from build123d import *

# Parameters (mm, degrees)
CROQUIS1_R                   = 15.000000000000002
SALIENTE_EXTRUIR1_DEPTH      = 8
CROQUIS2_R                   = 4.000000000000007
CROQUIS2_R_2                 = 1.4999999999999973
CORTAR_EXTRUIR1_DEPTH        = 3
SALIENTE_EXTRUIR2_START      = -4
SALIENTE_EXTRUIR2_DEPTH      = 4
SALIENTE_EXTRUIR3_DEPTH      = 10
SALIENTE_EXTRUIR3_DEPTH_BACK = 10
CROQUIS4_R                   = 1.999999999999995
CORTAR_EXTRUIR2_DEPTH        = 26.000000000000004
CROQUIS6_R                   = 1.499999999999999
CORTAR_EXTRUIR3_DEPTH        = 0.5


with BuildPart() as part:
    # Croquis1 → Saliente-Extruir1 (new body)
    with BuildSketch(Plane(origin=(3.102503887066035, -26.412068884743757, 0.2313913751144545), x_dir=(0.9931720445250996, 0.11665438489091776, -0.0010219880408017562), z_dir=(0.11665886153153528, -0.9931339327669669, 0.008700667387268338))):
        with Locations(Location((-115.80198834358447, 158.9846336736222, 0), (0, 0, 0.058557828))):
            Circle(CROQUIS1_R)
    extrude(amount=SALIENTE_EXTRUIR1_DEPTH)

    # Croquis2 → Cortar-Extruir1 (cut)
    with BuildSketch(Plane(origin=(4.03577477931832, -34.35714034687951, 0.3009967142126015), x_dir=(0.9931720445250996, 0.11665438489091778, -0.0010219880408017569), z_dir=(0.1166588615315353, -0.9931339327669669, 0.00870066738726834))):
        with Locations(Location((-115.8019883435845, 158.9846336736222, 0), (0, 0, 0.058557828))):
            Circle(CROQUIS2_R)
        with Locations(Location((-115.8019883435845, 168.9846336736222, 0), (0, 0, 0.058557828))):
            Circle(CROQUIS2_R_2)
        with Locations(Location((-115.8019883435845, 148.9846336736222, 0), (0, 0, 0.058557828))):
            Circle(CROQUIS2_R_2)
    extrude(amount=-CORTAR_EXTRUIR1_DEPTH, mode=Mode.SUBTRACT)

    # Croquis3 → Saliente-Extruir2 (add)
    with BuildSketch(Plane(origin=(4.03577477931832, -34.35714034687951, 0.3009967142126015), x_dir=(0.9931720445250996, 0.11665438489091778, -0.0010219880408017569), z_dir=(0.1166588615315353, -0.9931339327669669, 0.00870066738726834)).offset(SALIENTE_EXTRUIR2_START)):
        with BuildLine():
            Line((-140.80198834358453, 161.9846336736222), (-130.49892680028356, 161.9846336736222))
            ThreePointArc((-130.49892680028356, 161.98463367362223), (-129.9260267482204, 164.03552855912218), (-129.06848750500595, 165.98463367362243))
            Line((-129.0684875050059, 165.9846336736222), (-140.80198834358453, 165.9846336736222))
            Line((-140.80198834358453, 165.9846336736222), (-140.80198834358453, 161.9846336736222))
        make_face()
        with BuildLine():
            ThreePointArc((-129.06848750500598, 151.98463367362197), (-129.9260267482204, 153.9337387881222), (-130.49892680028356, 155.98463367362217))
            Line((-130.49892680028356, 155.9846336736222), (-140.80198834358453, 155.9846336736222))
            Line((-140.80198834358453, 155.9846336736222), (-140.80198834358453, 151.9846336736222))
            Line((-140.80198834358453, 151.9846336736222), (-129.06848750500592, 151.9846336736222))
        make_face()
        with BuildLine():
            Line((-125.01691169330087, 151.9846336736222), (-125.01691169330087, 155.9846336736222))
            Line((-125.01691169330087, 155.9846336736222), (-130.49892680028356, 155.9846336736222))
            ThreePointArc((-130.49892680028356, 155.98463367362217), (-129.9260267482204, 153.9337387881222), (-129.06848750500598, 151.98463367362197))
            Line((-129.06848750500592, 151.9846336736222), (-125.01691169330087, 151.9846336736222))
        make_face()
        with BuildLine():
            Line((-130.49892680028356, 161.9846336736222), (-125.01691169330087, 161.9846336736222))
            Line((-125.01691169330087, 161.9846336736222), (-125.01691169330087, 165.9846336736222))
            Line((-125.01691169330087, 165.9846336736222), (-129.0684875050059, 165.9846336736222))
            ThreePointArc((-129.06848750500595, 165.98463367362243), (-129.9260267482204, 164.03552855912218), (-130.49892680028356, 161.98463367362223))
        make_face()
    extrude(amount=SALIENTE_EXTRUIR2_DEPTH)

    # Croquis4 → Saliente-Extruir3 (add, two sides: drawn at the far end of the back side and taken through both)
    with BuildSketch(Plane(origin=(-6.683e-14, 1.3927822726245929, 158.97853283345188), x_dir=(1, 0, 4.2e-16), z_dir=(0, 0.008760483579084877, 0.9999616262274571)).offset(-SALIENTE_EXTRUIR3_DEPTH_BACK)):
        with Locations(Location((-134.05179749109138, -48.5645966599886, 0), (0, 0, 276.699314902))):
            Circle(CROQUIS4_R)
    extrude(amount=SALIENTE_EXTRUIR3_DEPTH + SALIENTE_EXTRUIR3_DEPTH_BACK)

    # Croquis5 → Cortar-Extruir2 (cut)
    with BuildSketch(Plane(origin=(-7.073e-14, 1.4803871084154419, 168.97814909572648), x_dir=(1, 0, 4.2e-16), z_dir=(0, 0.008760483579084877, 0.9999616262274571))):
        Polygon((-137.1921048729679, -53.52505022011607), (-133.51980518703422, -53.09369867037679), (-133.8184797680283, -50.5509407490388), (-135.80482385707867, -50.78425847210188), (-136.03814158014168, -48.79791438305168), (-136.2714593032048, -46.81157029400149), (-134.28511521415442, -46.578252570938396), (-134.47954467160224, -44.922982673441965), (-138.15184435753594, -45.35433422318124), align=None)
        with BuildLine():
            ThreePointArc((-136.03814158014154, -48.79791438305167), (-135.62133541037747, -47.32501982900029), (-134.28511521415442, -46.57825257093841))
            Line((-134.28511521415442, -46.578252570938396), (-136.2714593032048, -46.81157029400149))
            Line((-136.2714593032048, -46.81157029400149), (-136.03814158014168, -48.79791438305168))
        make_face()
        with BuildLine():
            ThreePointArc((-133.8184797680283, -50.550940749038816), (-135.2913743220797, -50.13413457927471), (-136.03814158014154, -48.79791438305167))
            Line((-136.03814158014168, -48.79791438305168), (-135.80482385707867, -50.78425847210188))
            Line((-135.80482385707867, -50.78425847210188), (-133.8184797680283, -50.5509407490388))
        make_face()
    extrude(amount=-CORTAR_EXTRUIR2_DEPTH, mode=Mode.SUBTRACT)

    # Croquis6 → Cortar-Extruir3 (cut)
    # profile 1 of 2: a face of its own
    with BuildSketch(Plane(origin=(4.03577477931832, -34.35714034687951, 0.3009967142126015), x_dir=(0.9931720445250996, 0.11665438489091778, -0.0010219880408017569), z_dir=(0.1166588615315353, -0.9931339327669669, 0.008700667387268341))):
        with BuildLine():
            Line((-111.32985238858495, 159.4846336736222), (-101.81091976395129, 159.4846336736222))
            ThreePointArc((-101.81091976395126, 159.48463367362265), (-112.97131478814173, 172.6954792792921), (-128.45109898425804, 164.9846336736222))
            Line((-128.45109898425804, 164.9846336736222), (-137.80198834358436, 164.98463367362217))
            Line((-137.80198834358436, 164.98463367362217), (-137.80198834358436, 162.98463367362217))
            Line((-137.80198834358436, 162.98463367362217), (-129.21839620858324, 162.9846336736222))
            ThreePointArc((-129.21839620858324, 162.9846336736222), (-129.6170142670406, 161.25290586501285), (-129.7930569232177, 159.48463367362226))
            Line((-129.7930569232177, 159.4846336736222), (-120.27412429858411, 159.4846336736222))
            ThreePointArc((-120.27412429858411, 159.48463367362217), (-115.80198834358455, 163.4846336736222), (-111.32985238858495, 159.48463367362223))
        make_face()
        with Locations(Location((-115.80198834358454, 168.9846336736222, 0), (0, 0, 0.058557828))):
            Circle(CROQUIS6_R, mode=Mode.SUBTRACT)
    # profile 2 of 2: a face of its own
    with BuildSketch(Plane(origin=(4.03577477931832, -34.35714034687951, 0.3009967142126015), x_dir=(0.9931720445250996, 0.11665438489091778, -0.0010219880408017569), z_dir=(0.1166588615315353, -0.9931339327669669, 0.008700667387268341))):
        with BuildLine():
            ThreePointArc((-128.45109898425804, 152.9846336736222), (-112.97131478814173, 145.2737880679523), (-101.81091976395126, 158.48463367362174))
            Line((-101.81091976395128, 158.4846336736222), (-111.32985238858495, 158.4846336736222))
            ThreePointArc((-111.32985238858495, 158.48463367362217), (-115.80198834358455, 154.4846336736222), (-120.27412429858411, 158.48463367362223))
            Line((-120.27412429858411, 158.4846336736222), (-129.7930569232177, 158.4846336736222))
            ThreePointArc((-129.7930569232177, 158.48463367362214), (-129.6170142670406, 156.71636148223155), (-129.21839620858327, 154.98463367362223))
            Line((-129.21839620858327, 154.98463367362223), (-137.80198834358436, 154.9846336736222))
            Line((-137.80198834358436, 154.9846336736222), (-137.80198834358436, 152.9846336736222))
            Line((-137.80198834358436, 152.9846336736222), (-128.45109898425804, 152.9846336736222))
        make_face()
        with Locations(Location((-115.80198834358453, 148.9846336736222, 0), (0, 0, 0.058557828))):
            Circle(CROQUIS6_R, mode=Mode.SUBTRACT)
    extrude(amount=-CORTAR_EXTRUIR3_DEPTH, mode=Mode.SUBTRACT)


solid = part.part
Could you check a few things on this model? Use its own coordinates, in mm. Coordinates: 2 decimals unless noted, no trailing zeros. Order: outer loops, then holes, each group sorted by start corner. A loop starts at its lowest first (then second) coordinate and runs counter-clockwise, first axis right, second up. Notation, with made-up numbers: (69, 26) - (99, 26) arc R20 cw to (99, 42) - close; hole circle Ø2 at (33, 17.5). An arc over 180 degrees is marked (long way). Answer in a Markdown table with one row per item. Add a question column.
(1) Will these pins go through, and if not, where does the flat tip stop? pin 1 (4 mm diameter, centred on x = -115.5, y = -44, fed in from +Z); pin 2 (1.5 mm diameter, centred on x = -126.5, z = 165.5, fed in from +Y); pin 3 (1.5 mm diameter, centred on x = -102.5, y = -41.5, fed in from -Z).
(2) I need wall thicknesses on L1, parallel to Z at x = -110.5, y = -45; L2, parallel to Y at x = -125, z = 159.5; L3, parallel to Y at x = -119, z = 156.5. Which ranges of each line are inside material? Lowest first, please.
(3) If we section it at A-A, the plane x = -129: Please give me the cut outline in (y, z), then the cut area to 3 significant figures.
(4) If we mould it in two halves opening along Y, with no side actions, what happens to faces 1 (the face through (-114.08, -45.32, 162.09)), 2 (the face through (-112.277, -44.785, 170.396))? For each: released by +Y, released by -Y, zero draft, split by the parting line, or undercut.
Results are:
| question | item | result |
|---|---|---|
| 1 | pin 1 | stops at z = 174.21 |
| 1 | pin 2 | stops at y = -44.13 |
| 1 | pin 3 | stops at z = 146.83 |
| 2 | L1 | z = 144.4 to 148.04, 150.74 to 155.44, 163.33 to 168.03, 170.75 to 174.37 |
| 2 | L2 | y = -48.12 to -40.06 |
| 2 | L3 | y = -46.94 to -39.39 |
| 3 | outline | (-48.65, 152.42) - (-44.62, 152.38) - (-44.59, 156.38) - (-48.62, 156.42) - (-48.63, 155.42) - (-48.12, 155.41) - (-48.14, 153.41) - (-48.64, 153.42) - close; (-48.56, 162.42) - (-44.54, 162.38) - (-44.5, 166.38) - (-48.53, 166.42) - (-48.54, 165.42) - (-48.03, 165.41) - (-48.05, 163.41) - (-48.56, 163.42) - close |
| 3 | area | 30.2 mm2 |
| 4 | face 1 | undercut |
| 4 | face 2 | undercut |
